```python
from build123d import *

# Parameters (mm, degrees)
BOSS_EXTRUDE1_START     = 22.3
BOSS_EXTRUDE1_DEPTH     = 30.9
CUT_EXTRUDE1_START      = 22.3
CUT_EXTRUDE1_DEPTH      = 29.7
BOSS_EXTRUDE2_START     = 22.3
BOSS_EXTRUDE2_DEPTH     = 1.2
CUT_EXTRUDE2_START      = 22.2
SKETCH4_W               = 50.6
SKETCH4_H               = 74.3
CUT_EXTRUDE2_DEPTH      = 1.4
CUT_EXTRUDE3_START      = 22.2
SKETCH5_W               = 60.6
SKETCH5_H               = 8.3
CUT_EXTRUDE3_DEPTH      = 1.4
BOSS_EXTRUDE3_START     = 29
SKETCH6_R               = 3.5
BOSS_EXTRUDE3_DEPTH     = 23
CUT_EXTRUDE4_DEPTH      = 87.278212777
CUT_EXTRUDE4_DEPTH_BACK = 87.278212777
SKETCH7_R               = 1.725
CUT_EXTRUDE5_START      = 47.2
CUT_EXTRUDE5_DEPTH      = 6.1


with BuildPart() as part:
    # Sketch1 → Boss-Extrude1 (new body)
    with BuildSketch(Plane.XY.offset(BOSS_EXTRUDE1_START)):
        Polygon((-43.7, 0), (-43.162, -6.8362), (-41.5612, -13.504), (-31.6, -50), (31.6, -50), (41.5612, -13.504), (43.162, -6.8362), (43.7, 0), (43.162, 6.8362), (41.5612, 13.504), (38.937, 19.8394), (35.354, 25.6862), (30.9006, 30.9006), (25.6862, 35.354), (19.8394, 38.937), (13.504, 41.5612), (6.8362, 43.162), (0, 43.7), (-6.8362, 43.162), (-13.504, 41.5612), (-19.8394, 38.937), (-25.6862, 35.354), (-30.9006, 30.9006), (-35.354, 25.6862), (-38.937, 19.8394), (-41.5612, 13.504), (-43.162, 6.8362), align=None)
    extrude(amount=BOSS_EXTRUDE1_DEPTH)

    # Sketch2 → Cut-Extrude1 (cut)
    with BuildSketch(Plane.XY.offset(CUT_EXTRUDE1_START)):
        Polygon((-42.5, 0), (-41.9768, -6.6485), (-40.4199, -13.1332), (-30.4, -52), (30.4, -52), (40.4199, -13.1332), (41.9768, -6.6485), (42.5, 0), (41.9768, 6.6485), (40.4199, 13.1332), (37.8678, 19.2946), (34.3832, 24.9809), (30.052, 30.052), (24.9809, 34.3832), (19.2946, 37.8678), (13.1332, 40.4199), (6.6485, 41.9768), (0, 42.5), (-6.6485, 41.9768), (-13.1332, 40.4199), (-19.2946, 37.8678), (-24.9809, 34.3832), (-30.052, 30.052), (-34.3832, 24.9809), (-37.8678, 19.2946), (-40.4199, 13.1332), (-41.9768, 6.6485), align=None)
    extrude(amount=CUT_EXTRUDE1_DEPTH, mode=Mode.SUBTRACT)

    # Sketch3 → Boss-Extrude2 (add)
    with BuildSketch(Plane.XY.offset(BOSS_EXTRUDE2_START)):
        Polygon((-42.5, 0), (-41.9768, -6.6485), (-40.4199, -13.1332), (-30.4, -52), (30.4, -52), (40.4199, -13.1332), (41.9768, -6.6485), (42.5, 0), (41.9768, 6.6485), (40.4199, 13.1332), (37.8678, 19.2946), (34.3832, 24.9809), (30.052, 30.052), (24.9809, 34.3832), (19.2946, 37.8678), (13.1332, 40.4199), (6.6485, 41.9768), (0, 42.5), (-6.6485, 41.9768), (-13.1332, 40.4199), (-19.2946, 37.8678), (-24.9809, 34.3832), (-30.052, 30.052), (-34.3832, 24.9809), (-37.8678, 19.2946), (-40.4199, 13.1332), (-41.9768, 6.6485), align=None)
    extrude(amount=BOSS_EXTRUDE2_DEPTH)

    # Sketch4 → Cut-Extrude2 (cut)
    with BuildSketch(Plane.XY.offset(CUT_EXTRUDE2_START)):
        with Locations((0, -15.85)):
            Rectangle(SKETCH4_W, SKETCH4_H)
    extrude(amount=CUT_EXTRUDE2_DEPTH, mode=Mode.SUBTRACT)

    # Sketch5 → Cut-Extrude3 (cut)
    with BuildSketch(Plane.XY.offset(CUT_EXTRUDE3_START)):
        with Locations((0, -48.85)):
            Rectangle(SKETCH5_W, SKETCH5_H)
    extrude(amount=CUT_EXTRUDE3_DEPTH, mode=Mode.SUBTRACT)

    # Sketch6 → Boss-Extrude3 (add)
    with BuildSketch(Plane.XY.offset(BOSS_EXTRUDE3_START)):
        with Locations((5, 14.35)):
            Circle(SKETCH6_R)
        with Locations((-5, -34.65)):
            Circle(SKETCH6_R)
    extrude(amount=BOSS_EXTRUDE3_DEPTH)

    # Sketch7 → Cut-Extrude4 (cut, two sides: drawn at the far end of the back side and taken through both)
    with BuildSketch(Plane.XY.offset(-CUT_EXTRUDE4_DEPTH_BACK)):
        with Locations((5, 14.35)):
            Circle(SKETCH7_R)
        with Locations((-5, -34.65)):
            Circle(SKETCH7_R)
    extrude(amount=CUT_EXTRUDE4_DEPTH + CUT_EXTRUDE4_DEPTH_BACK, mode=Mode.SUBTRACT)

    # Sketch8 → Cut-Extrude5 (cut)
    with BuildSketch(Plane.XY.offset(CUT_EXTRUDE5_START)):
        Polygon((7.8, 15.966580754), (5, 17.583161507), (2.2, 15.966580754), (2.2, 12.733419246), (5, 11.116838493), (7.8, 12.733419246), align=None)
        Polygon((-2.2, -33.033419246), (-5, -31.416838493), (-7.8, -33.033419246), (-7.8, -36.266580754), (-5, -37.883161507), (-2.2, -36.266580754), align=None)
    extrude(amount=CUT_EXTRUDE5_DEPTH, mode=Mode.SUBTRACT)


solid = part.part
```
Geometry: final body of the model. Coordinates: model frame, mm. A direction names the side the tool comes from. Coordinates: 2 decimals unless noted, no trailing zeros. Loops run counter-clockwise (first coordinate to the right, second up) from the corner with the lowest first, then second, coordinate; pieces in that order, holes last. Notation, with made-up numbers: (-11.5, 4) -> (3.5, 4) arc R12 cw to (3.5, 20) -> close; hole circle Ø2 at (-14.5, 29.5). An arc over 180 degrees is marked (long way). Use a Markdown table: item, result. Add a question column.
(1) Section query B-B, the plane z = 35. State how many separate pieces and enclosed holes the cut face has, plus the area to 3 significant figures.
(2) Section query A-A, the plane y = -34.65. Return loops of the section in (x, z) (3 decimals), plus the area to 3 significant figures.
(3) Line query: line 1 along X through (y, z) = (-37, 46.5); line 2 along Z through (x, y) = (-23, 26); line 3 along X through (y, z) = (12, 38). Output: solid intervals per line, ascending.
(4) Pin query (flat end, axial travel): pin 1 Ø1.7 at (x, y) = (4.5, 15) entering from +Z; pin 2 Ø1 at (y, z) = (-34, 51.5) entering from -X; pin 3 Ø2.5 at (y, z) = (15, 50.5) entering from -X; pin 4 Ø5.5 at (x, y) = (-3.5, -33) entering from -Z. Return the tip coordinate at first contact, or that it passes through.
(5) Mould query, pull axis Z, two halves, no side actions, for faces 4 (the flat face through (35.601, -31.825, 37.55)), 5 (the flat face through (3, 14, 29)), 6 (the flat face through (43.435, 3.37, 37.534)). Classes: pulls with the +Z half, pulls with the -Z half, needs draft (parallel to the pull), parting line crosses it, or undercut.
(6) Access query for faces 1 (the flat face through (-39.126, 16.257, 37.55)), 2 (the flat face through (3.466, 43.427, 37.534)), 3 (the flat face through (6.38, 11.914, 50.158)). Directions: +Z, -Z, +X, -X, +Y, -Y. A direction counts if a zero-diameter tool reaches every point of the face in a straight line with its end or side. Return the directions, or none.
Answer:
| question | item | result |
|---|---|---|
| 1 | separate pieces | 3 |
| 1 | enclosed holes | 2 |
| 1 | area | 323 mm^2 |
| 2 | outline | (-35.79, 22.3) -> (-25.3, 22.3) -> (-25.3, 23.5) -> (-34.873, 23.5) -> (-34.873, 52) -> (-8.5, 52) -> (-8.5, 29) -> (-6.725, 29) -> (-6.725, 47.2) -> (-7.8, 47.2) -> (-7.8, 53.2) -> (-35.79, 53.2) -> close; (-3.275, 29) -> (-1.5, 29) -> (-1.5, 52) -> (34.873, 52) -> (34.873, 23.5) -> (25.3, 23.5) -> (25.3, 22.3) -> (35.79, 22.3) -> (35.79, 53.2) -> (-2.2, 53.2) -> (-2.2, 47.2) -> (-3.275, 47.2) -> close |
| 2 | area | 228 mm^2 |
| 3 | line 1 | x = -35.15 to -34.27, -7.59 to -2.41, 34.27 to 35.15 |
| 3 | line 2 | z = 22.3 to 23.5, 52 to 53.2 |
| 3 | line 3 | x = -41.92 to -40.69, 2.41 to 7.59, 40.69 to 41.92 |
| 4 | pin 1 | passes through |
| 4 | pin 2 | stops at x = -36.1 |
| 4 | pin 3 | stops at x = -41.46 |
| 4 | pin 4 | stops at z = 29 |
| 5 | face 4 | undercut |
| 5 | face 5 | pulls with the -Z half |
| 5 | face 6 | needs draft |
| 6 | face 1 | none |
| 6 | face 2 | +Z, -Z, +X, +Y |
| 6 | face 3 | +Z |
